Verification items for this drawing (mm, ordinates from the low corner). A direction names the side the tool comes from. Round coordinates to 2 decimals unless told otherwise and drop trailing zeros. Order: outer loops, then holes, each group sorted by start corner. A loop starts at its lowest first (then second) coordinate and runs counter-clockwise, first axis right, second up. Notation, with made-up numbers: (-32, -12) -> (16, -12) arc R16 cw to (16, -1) -> close; hole circle Ø10 at (-29, -26.5). An arc over 180 degrees is marked (long way). Return JSON: item names as keys, results as strings. Group by question number.
Item 1: Sectioned sample at D-D on y = 9. Record the cut outline in (x, z), plus the area to 3 significant figures.
Item 2: Sectioned sample at C-C on x = 18. Record the cut outline in (y, z).
Item 3: Depth check by flat-ended pin: pin 1 Ø5 at (x, y) = (7, 4) entering from +Z; pin 2 Ø3.5 at (y, z) = (6.5, 5.5) entering from +X; pin 3 Ø2.5 at (x, y) = (18, 5) entering from -Z. Enter the tip coordinate at first touch or a pass-through.
Item 4: Sectioned sample at A-A on y = 5. Record the cut outline in (x, z).
Item 5: Sectioned sample at B-B on z = 21. Record the cut outline in (x, y).
Item 6: Access from +Z, -Z, +X, -X, +Y, -Y to the whole of each face (thin tool, end or side, straight path). Record for the marked faces 1, 2, 3, 4 and 5.
Item 7: Scan lines: probe 1 along Z at (x, y) = (15, 1.75); probe 2 along Y at (x, z) = (18, 42.4); probe 3 along Z at (x, y) = (4, 6.5). Record each from-to range of solid material in increasing order. Write a range as from..to.
Item 8: Draft check along Z on the marked faces 6, 7 and 8. Enter one of: pulls with the +Z half, pulls with the -Z half, needs draft (parallel to the pull), parting line crosses it, or undercut.
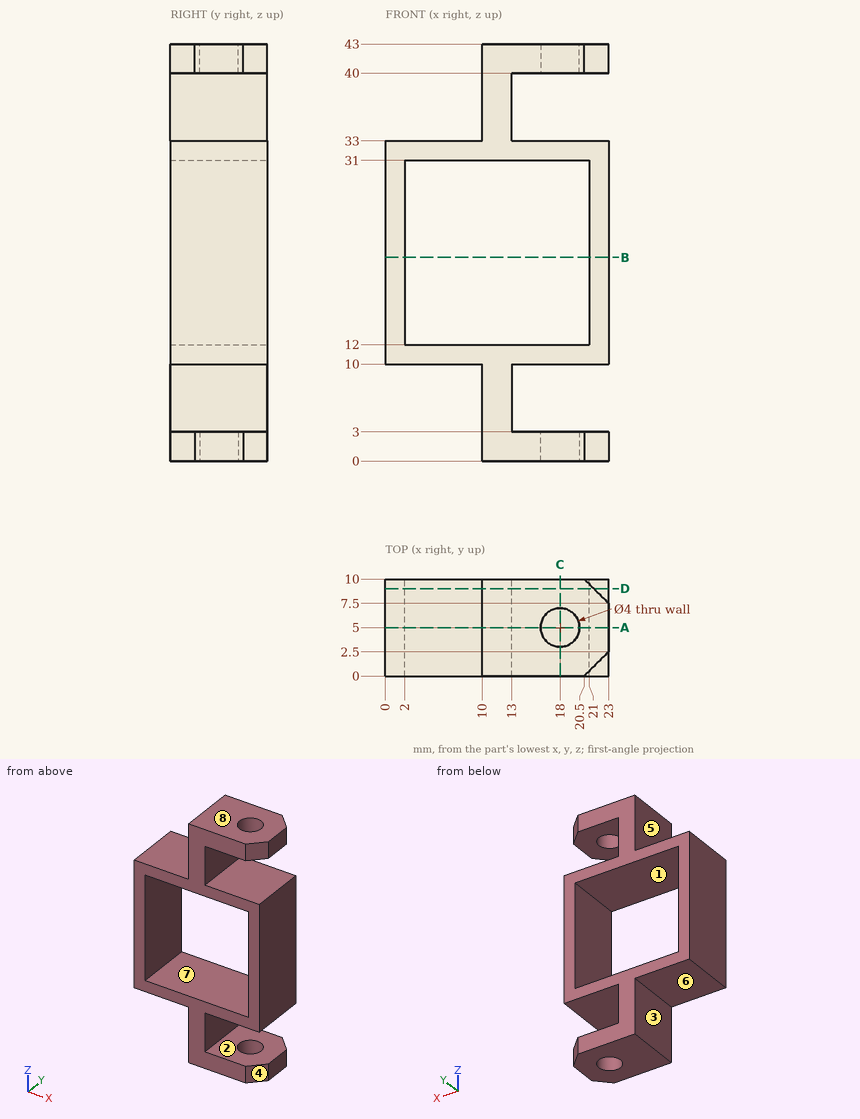
Recorded:
{
 "1": {"outline": "(0, 10) -> (10, 10) -> (10, 0) -> (21.5, 0) -> (21.5, 3) -> (13, 3) -> (13, 10) -> (23, 10) -> (23, 33) -> (13, 33) -> (13, 40) -> (21.5, 40) -> (21.5, 43) -> (10, 43) -> (10, 33) -> (0, 33) -> close; hole (2, 12) -> (21, 12) -> (21, 31) -> (2, 31) -> close", "area": "279 mm²"},
 "2": {"outline": "(0, 0) -> (3, 0) -> (3, 3) -> (0, 3) -> close; (0, 10) -> (10, 10) -> (10, 12) -> (0, 12) -> close; (0, 31) -> (10, 31) -> (10, 33) -> (0, 33) -> close; (0, 40) -> (3, 40) -> (3, 43) -> (0, 43) -> close; (7, 0) -> (10, 0) -> (10, 3) -> (7, 3) -> close; (7, 40) -> (10, 40) -> (10, 43) -> (7, 43) -> close"},
 "3": {"pin 1": "z = 33", "pin 2": "x = 13", "pin 3": "z = 10"},
 "4": {"outline": "(0, 10) -> (10, 10) -> (10, 0) -> (16, 0) -> (16, 3) -> (13, 3) -> (13, 10) -> (23, 10) -> (23, 33) -> (13, 33) -> (13, 40) -> (16, 40) -> (16, 43) -> (10, 43) -> (10, 33) -> (0, 33) -> close; (20, 0) -> (23, 0) -> (23, 3) -> (20, 3) -> close; (20, 40) -> (23, 40) -> (23, 43) -> (20, 43) -> close; hole (2, 12) -> (21, 12) -> (21, 31) -> (2, 31) -> close"},
 "5": {"outline": "(0, 0) -> (2, 0) -> (2, 10) -> (0, 10) -> close; (21, 0) -> (23, 0) -> (23, 10) -> (21, 10) -> close"},
 "6": {"face 1": "+Y, -Y", "face 2": "+X, +Y, -Y", "face 3": "-Z, -X, +Y, -Y", "face 4": "-Z, +X, -Y", "face 5": "+Z, -X, +Y, -Y"},
 "7": {"probe 1": "0..3, 10..12, 31..33, 40..43", "probe 2": "0..3, 7..10", "probe 3": "10..12, 31..33"},
 "8": {"face 6": "pulls with the -Z half", "face 7": "undercut", "face 8": "pulls with the +Z half"}
}
